from build123d import *

# Parameters (mm, degrees)
F0_R     = 1.5875
F1_DEPTH = 3.175


with BuildPart() as f1:
    # F0 (on Top) → F1 (new body)
    with BuildSketch(Plane.XY):
        with BuildLine():
            ThreePointArc((-5.398182, 26.445581), (-4.837228, 26.553914), (-4.274107, 26.65035))
            ThreePointArc((-4.274107, 26.65035), (-2.26211, 30.204549), (-5.398182, 32.820944))
            ThreePointArc((-5.398182, 32.820944), (-24.789003, 24.789003), (-32.820944, 5.398182))
            ThreePointArc((-32.820944, 5.398182), (-30.204549, 2.26211), (-26.65035, 4.274107))
            ThreePointArc((-26.65035, 4.274107), (-26.553914, 4.837228), (-26.445581, 5.398182))
            ThreePointArc((-26.445581, 5.398182), (-19.085454, 19.085454), (-5.398182, 26.445581))
        make_face()
        with Locations((-8.573182, 29.633263)):
            Circle(F0_R, mode=Mode.SUBTRACT)
    extrude(amount=-F1_DEPTH)


solid = f1.part
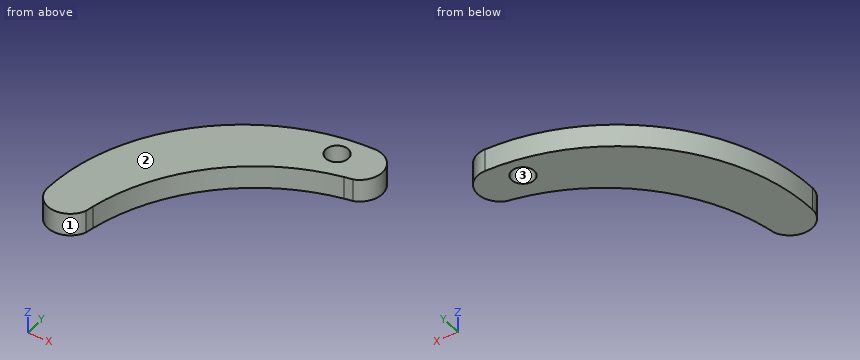
The model under review builds one solid part; all positions refer to its coordinate system, in mm. Face numbers are marked on the shaded views. Round coordinates to 2 decimals unless told otherwise and drop trailing zeros. Write each loop counter-clockwise with the first axis right and the second up, starting at its lowest first coordinate (ties: lowest second). Pieces come first, ordered by that corner, then holes. Notation, with made-up numbers: M -32,-9.75 L 2,-9.75 A20 cw 2,21.25 Z; hole C -21,-18.75 d10. An arc over 180 degrees is marked long. Use a Markdown table: item, result. Add a question column.
Q1. We need section C-C, the plane x = -16. State the section outline as (y, z) points (3 decimals).
Q2. Insertion check: pin 1 (1.5 mm diameter, centred on x = -21.5, z = -3, fed in from +Y); pin 2 (1 mm diameter, centred on x = -22.5, z = -1.5, fed in from -Y); pin 3 (3 mm diameter, centred on x = -24.5, y = 29, fed in from -Z). Each pin has a flat end and moves straight along its axis. Give the tip position at first contact, or say it passes through.
Q3. We need section A-A, the plane z = -2.8. State the section outline as (x, y) points (1 decimal).
Q4. The part is to be moulded in two halves that separate along X. For the marked faces 1, 2 and 3, say which applies: pulls with the +X half, pulls with the -X half, needs draft (parallel to the pull), parting line crosses it, or undercut.
Q5. To check wall thickness, follow line 1 (X direction, y = 30.5, z = -1.35); line 2 (X direction, y = 4, z = -2.95); line 3 (Y direction, x = -18, z = -2.8). State the ranges of each line that lie inside material, in increasing order.
Q6. We need section B-B, the plane y = 21. State the section outline as (x, z) points (3 decimals).
Findings below:
| question | item | result |
|---|---|---|
| 1 | outline | M 21.737,-3.175 L 30.689,-3.175 L 30.689,0 L 21.737,0 Z |
| 2 | pin 1 | stops at y = 28.12 |
| 2 | pin 2 | stops at y = 14.12 |
| 2 | pin 3 | passes through |
| 3 | outline | M -32.8,5.4 A3.2 ccw -26.7,4.3 A27 cw -26.4,5.4 A27 cw -5.4,26.4 A27 cw -4.3,26.7 A3.2 ccw -5.4,32.8 A27.4 ccw Z; hole C -8.6,29.6 d3.2 |
| 4 | face 1 | parting line crosses it |
| 4 | face 2 | needs draft |
| 4 | face 3 | undercut |
| 5 | line 1 | x = -16.44 to -9.9, -7.24 to -2.33 |
| 5 | line 2 | x = -32.5 to -26.77 |
| 5 | line 3 | y = 20.11 to 29.75 |
| 6 | outline | M -27.95,-3.175 L -16.956,-3.175 L -16.956,0 L -27.95,0 Z |
